from build123d import *

# Parameters (mm, degrees)
SKETCH1_R           = 0.5
BOSS_EXTRUDE1_DEPTH = 0.762


with BuildPart() as part:
    # Sketch1 → Boss-Extrude1 (new body)
    with BuildSketch(Plane.XY):
        with BuildLine():
            Line((-1.1811, -1.060735141), (-1.1811, -7.829264859))
            ThreePointArc((-1.1811, -7.829264859), (0, -10.4775), (1.1811, -7.829264859))
            Line((1.1811, -7.829264859), (1.1811, -1.060735141))
            ThreePointArc((1.1811, -1.060735141), (1.5875, 0), (1.1811, 1.060735141))
            Line((1.1811, 1.060735141), (1.1811, 16.51))
            Line((1.1811, 16.51), (0, 19.685))
            Line((0, 19.685), (-1.1811, 16.51))
            Line((-1.1811, 16.51), (-1.1811, 1.060735141))
            ThreePointArc((-1.1811, 1.060735141), (-1.5875, 0), (-1.1811, -1.060735141))
        make_face()
        Circle(SKETCH1_R, mode=Mode.SUBTRACT)
    extrude(amount=BOSS_EXTRUDE1_DEPTH)


solid = part.part
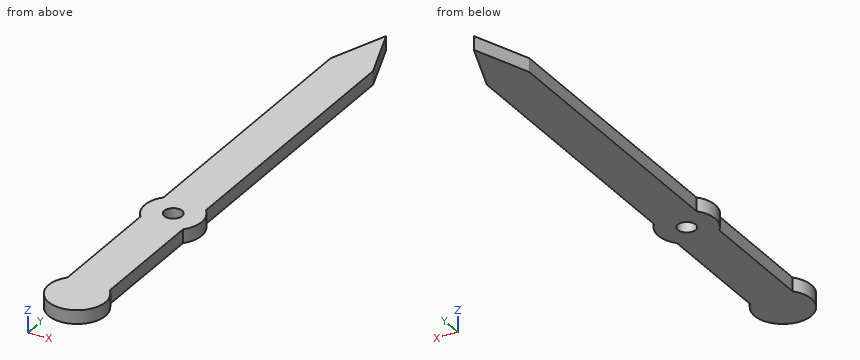
Geometry: final body of the model. Coordinates: model frame, mm. Round coordinates to 2 decimals unless told otherwise and drop trailing zeros. Loops run counter-clockwise (first coordinate to the right, second up) from the corner with the lowest first, then second, coordinate; pieces in that order, holes last.
Q1. Section B-B on z = 0.5. Return loops of the section in (x, y) (1 decimal).
Q2. Section A-A on y = 0. Return loops of the section in (x, z), plus the area to 3 significant figures.
Q3. Section D-D on y = 13. Return loops of the section in (x, z), plus the area to 3 significant figures.
Q4. Material intervals for L1, parallel to X at y = 14.5, z = 0.25; L2, parallel to X at y = -9, z = 0.6, sorted ascending.
Q5. Section C-C on x = -0.25. Return loops of the section in (y, z).
Evaluation:
1. outline: (-1.2, -7.8) arc R1.6 ccw (long way) to (1.2, -7.8) - (1.2, -1.1) arc R1.6 ccw to (1.2, 1.1) - (1.2, 16.5) - (0, 19.7) - (-1.2, 16.5) - (-1.2, 1.1) arc R1.6 ccw to (-1.2, -1.1) - close; hole circle Ø1 at (0, 0)
2. outline: (-1.59, 0) - (-0.5, 0) - (-0.5, 0.76) - (-1.59, 0.76) - close; (0.5, 0) - (1.59, 0) - (1.59, 0.76) - (0.5, 0.76) - close
2. area: 1.66 mm2
3. outline: (-1.18, 0) - (1.18, 0) - (1.18, 0.76) - (-1.18, 0.76) - close
3. area: 1.80 mm2
4. L1: x = -1.18 to 1.18
4. L2: x = -1.58 to 1.58
5. outline: (-10.46, 0) - (-0.43, 0) - (-0.43, 0.76) - (-10.46, 0.76) - close; (0.43, 0) - (19.01, 0) - (19.01, 0.76) - (0.43, 0.76) - close
